from build123d import *

# Parameters (mm, degrees)
F0_W     = 30
F0_H     = 30
F1_DEPTH = 36
F2_R     = 13.5
F3_DEPTH = 20
F4_SIZE  = 5
F5_R     = 1


with BuildPart() as f1:
    # F0 (on Top) → F1 (new body)
    with BuildSketch(Plane.XY):
        Rectangle(F0_W, F0_H)
    extrude(amount=F1_DEPTH)

    # F2 (on Top) → F3 (join)
    with BuildSketch(Plane.XY):
        Circle(F2_R)
    extrude(amount=-F3_DEPTH)

    # F4
    f4_edges = [f1.edges().sort_by_distance(p)[0] for p in [
        (-13.5, 0, -20),
    ]]
    chamfer(f4_edges, length=F4_SIZE)

    # F5
    f5_edges = [f1.edges().sort_by_distance(p)[0] for p in [
        (0, -15, 0),
        (-15, 0, 0),
        (0, 15, 0),
        (15, 0, 0),
        (15, -15, 18),
        (-15, -15, 18),
        (-15, 15, 18),
        (15, 15, 18),
        (0, -15, 36),
        (-15, 0, 36),
        (15, 0, 36),
        (0, 15, 36),
    ]]
    fillet(f5_edges, radius=F5_R)


solid = f1.part
Verification items for the finished model (mm, model axes). A direction names the side the tool comes from. Coordinates: 2 decimals unless noted, no trailing zeros. Write each loop counter-clockwise with the first axis right and the second up, starting at its lowest first coordinate (ties: lowest second). Pieces come first, ordered by that corner, then holes. Notation, with made-up numbers: M 13,-19.75 L 50,-19.75 A22 cw 50,2.25 Z; hole C -35,12 d3. An arc over 180 degrees is marked long. Use a Markdown table: item, result.
Q1. Sectioned sample at A-A, the plane y = 0. Record the boundary of the cut face in (x, z), plus the area to 3 significant figures.
Reply:
| item | result |
|---|---|
| outline | M -15,1 A1 ccw -14,0 L -13.5,0 L -13.5,-15 L -8.5,-20 L 8.5,-20 L 13.5,-15 L 13.5,0 L 14,0 A1 ccw 15,1 L 15,35 A1 ccw 14,36 L -14,36 A1 ccw -15,35 Z |
| area | 1,590 mm² |
Q2. Thickness scan on line 1 (Z direction, x = 9.25, y = -12); line 2 (Z direction, x = 10, y = 6.75); line 3 (X direction, y = 2, z = -11). Record the ranges inside material, lowest first.
Reply:
| item | result |
|---|---|
| line 1 | z = 0 to 36 |
| line 2 | z = -16.44 to 36 |
| line 3 | x = -13.35 to 13.35 |
Q3. Sectioned sample at C-C, the plane z = -10.5. Record the boundary of the cut face in (x, y).
Reply:
| item | result |
|---|---|
| outline | C 0,0 d27 |
Q4. Go/stop test with flat-tipped pins: P1, Ø3, axis at y = -5.5, z = -12.5, coming from the +X side; P2, Ø5, axis at x = 6, y = 10, coming from the -Z side. Record where each tip stops, or that it passes through.
Reply:
| item | result |
|---|---|
| P1 | stops at x = 12.89 |
| P2 | stops at z = -19.34 |
Q5. Set-up check for faces 1 (the face through (-2.93, -13.18, -7.4)), 2 (the face through (0, 0, -20)): record each of +Z, -Z, +X, -X, +Y, -Y from which the full face is reachable in a straight line by a thin tool's end or side.
Reply:
| item | result |
|---|---|
| face 1 | -Z |
| face 2 | -Z, +X, -X, +Y, -Y |
